Check sheet for the drawn part. Datum: minimum x, y, z corner. Units: mm. A direction names the side the tool comes from. Give positions to 0.01 mm unless a question says otherwise; leave off trailing zeros. Order: outer loops, then holes, each group sorted by start corner. A loop starts at its lowest first (then second) coordinate and runs counter-clockwise, first axis right, second up. Notation, with made-up numbers: M 34.5,69 L 66.5,69 A21 cw 66.5,95 Z; hole C -30,17 d7. An arc over 180 degrees is marked long. Put each result on its own line as item: value. Start each with the question number.
Q1. Section check D-D on x = 65. Record the cut outline in (y, z).
Q2. Go/stop test with flat-tipped pins: pin 1 (5 mm diameter, centred on x = 23.5, y = 4, fed in from -Z); pin 2 (5 mm diameter, centred on x = 71, y = 6, fed in from +Z). Record where each tip stops, or that it passes through.
Q3. Section check A-A on z = 26.5. Record the cut outline in (x, y), then the cut area to 3 significant figures.
Q4. Section check C-C on y = 9. Record the cut outline in (x, z), then the cut area to 3 significant figures.
Q5. Material ranges on L1, parallel to X at y = 5.5, z = 39.5; L2, parallel to Z at x = 7, y = 1; L3, parallel to Z at x = 38.5, y = 8.5 (1 decimal), recorded low to high.
Q6. Access from +Z, -Z, +X, -X, +Y, -Y to the whole of each face (thin tool, end or side, straight path). Record for the marked faces 4, 5, 6 and 7.
Q7. Section check B-B on x = 6.5. Record the cut outline in (y, z).
Q8. Mould release check, pull along X, two halves, no side actions. Record for the marked faces 1, 2 and 3: +X half, -X half, draft (parallel to the pull), parting line (faces both ways), or undercut.
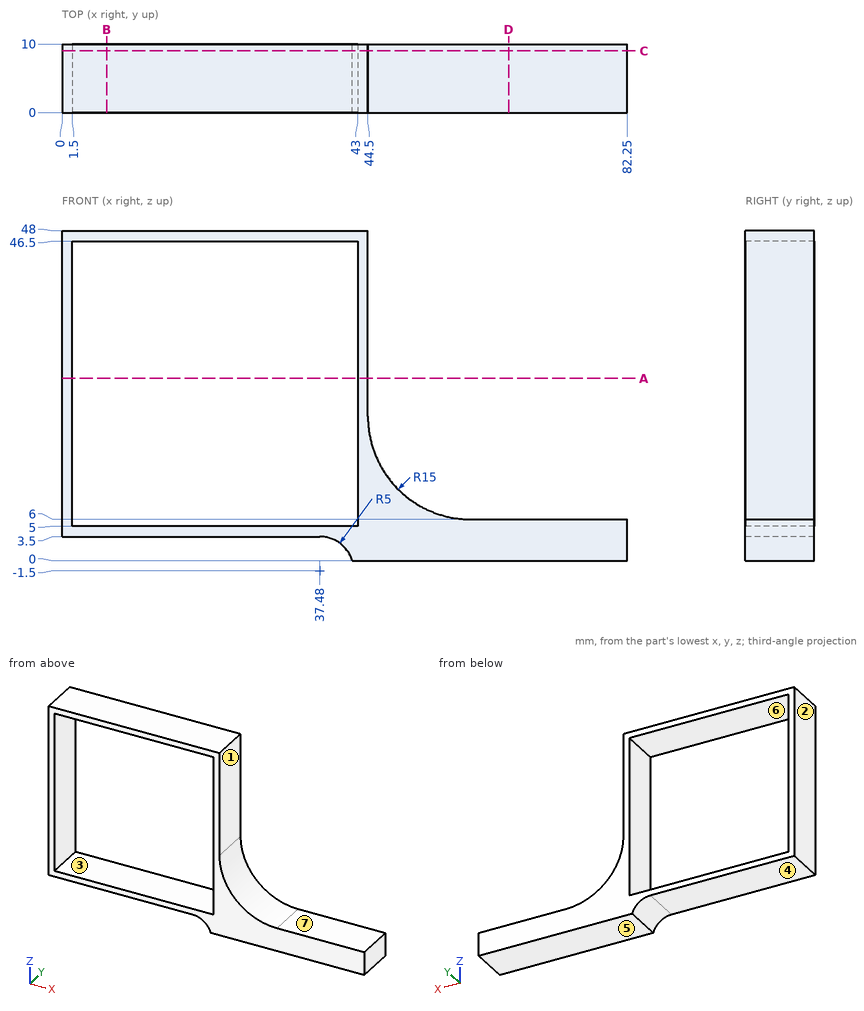
Results found:
1. outline: M 0,0 L 10,0 L 10,6 L 0,6 Z
2. pin 1: stops at z = 3.5
2. pin 2: stops at z = 6
3. outline: M 0,0 L 1.5,0 L 1.5,10 L 0,10 Z; M 43,0 L 44.5,0 L 44.5,10 L 43,10 Z
3. area: 30.0 mm^2
4. outline: M 0,3.5 L 37.48,3.5 A5 cw 42.25,0 L 82.25,0 L 82.25,6 L 59.5,6 A15 cw 44.5,21 L 44.5,48 L 0,48 Z; hole M 1.5,5 L 43,5 L 43,46.5 L 1.5,46.5 Z
4. area: 545 mm^2
5. L1: x = 0 to 1.5, 43 to 44.5
5. L2: z = 3.5 to 5, 46.5 to 48
5. L3: z = 3.4 to 5, 46.5 to 48
6. face 4: -Z, -X, +Y, -Y
6. face 5: -Z, +X, -X, +Y, -Y
6. face 6: +Y, -Y
6. face 7: +Z, +X, +Y, -Y
7. outline: M 0,3.5 L 10,3.5 L 10,5 L 0,5 Z; M 0,46.5 L 10,46.5 L 10,48 L 0,48 Z
8. face 1: +X half
8. face 2: -X half
8. face 3: undercut
